Source: three-view drawing plus pictorial views. Frame: mm from the lowest corner of the part. Give positions to 0.01 mm unless a question says otherwise; leave off trailing zeros. Order: outer loops, then holes, each group sorted by start corner. A loop starts at its lowest first (then second) coordinate and runs counter-clockwise, first axis right, second up. Notation, with made-up numbers: (28, -35.75) - (81, -35.75) arc R26 ccw to (81, -10.75) - close; hole circle Ø2 at (6, 73). An arc over 180 degrees is marked (long way). Answer in a Markdown table with one row per item. Add a question column.
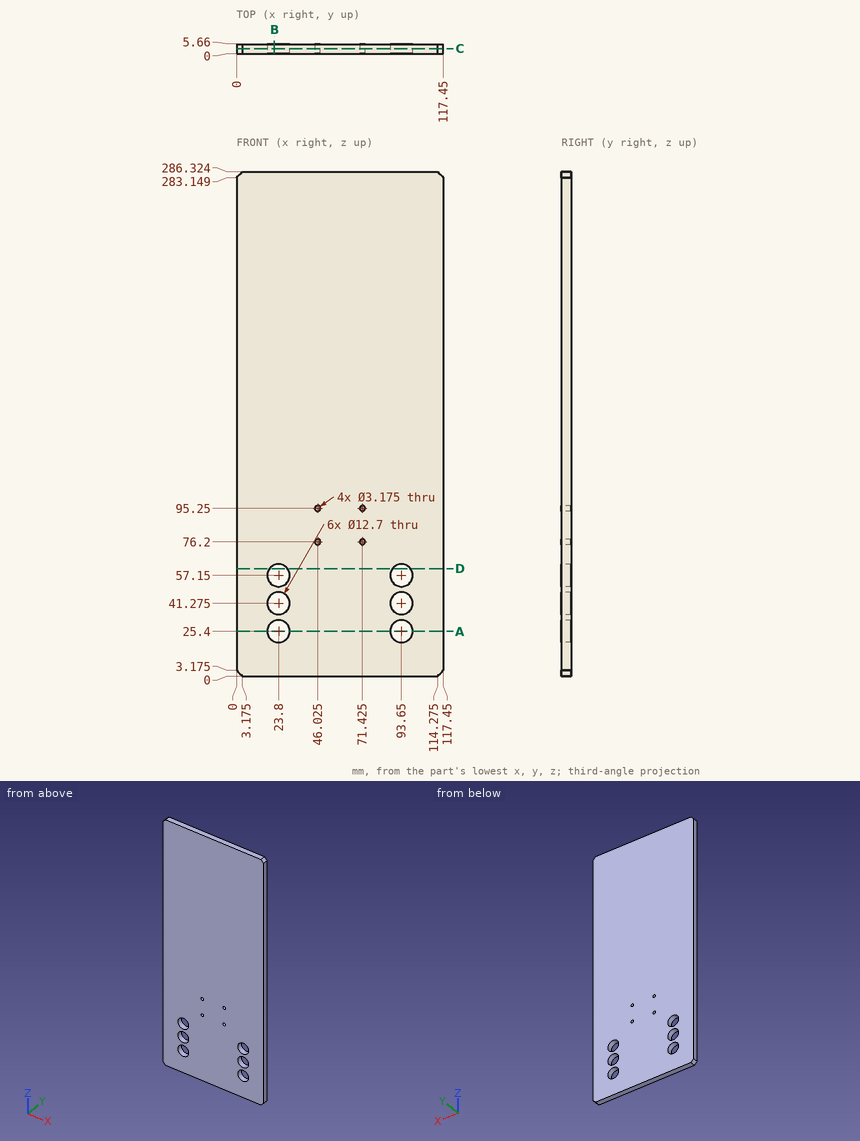
Q1. Contact query for a flat-ended pin moving along its axis: P1, Ø10, axis at x = 93.65, z = 41.28, coming from the -Y side. Output: stop coordinate, or through.
Q2. Section A-A, the plane z = 25.4. Return loops of the section in (x, y).
Q3. Line query: probe 1 along Z at (x, y) = (19, 4.3); probe 2 along Z at (x, y) = (45.5, 3.9); probe 3 along Z at (x, y) = (28, 0.8). Output: solid intervals per line, ascending.
Q4. Section C-C, the plane y = 3.05. State how many separate pieces and enclosed holes the cut face has, then the cut area to 3 significant figures.
Q5. Section B-B, the plane x = 21.5. Return loops of the section in (y, z).
Q6. Section D-D, the plane z = 61. Return loops of the section in (x, y).
Computed:
| question | item | result |
|---|---|---|
| 1 | P1 | passes through |
| 2 | outline | (0, 0) - (17.45, 0) - (17.45, 5.66) - (0, 5.66) - close; (30.15, 0) - (87.3, 0) - (87.3, 5.66) - (30.15, 5.66) - close; (100, 0) - (117.45, 0) - (117.45, 5.66) - (100, 5.66) - close |
| 3 | probe 1 | z = 0 to 21.24, 29.56 to 37.12, 45.43 to 52.99, 61.31 to 286.32 |
| 3 | probe 2 | z = 0 to 74.7, 77.7 to 93.75, 96.75 to 286.32 |
| 3 | probe 3 | z = 0 to 20.64, 30.16 to 36.51, 46.04 to 52.39, 61.91 to 286.32 |
| 4 | separate pieces | 1 |
| 4 | enclosed holes | 10 |
| 4 | area | 32,800 mm^2 |
| 5 | outline | (0, 0) - (5.66, 0) - (5.66, 19.48) - (0, 19.48) - close; (0, 31.32) - (5.66, 31.32) - (5.66, 35.36) - (0, 35.36) - close; (0, 47.19) - (5.66, 47.19) - (5.66, 51.23) - (0, 51.23) - close; (0, 63.07) - (5.66, 63.07) - (5.66, 286.32) - (0, 286.32) - close |
| 6 | outline | (0, 0) - (18.75, 0) - (18.75, 5.66) - (0, 5.66) - close; (28.85, 0) - (88.6, 0) - (88.6, 5.66) - (28.85, 5.66) - close; (98.7, 0) - (117.45, 0) - (117.45, 5.66) - (98.7, 5.66) - close |
